Job drawing, mm, ordinate dimensions from the low corner. One solid piece. Give positions to 0.01 mm unless a question says otherwise; leave off trailing zeros. Order: outer loops, then holes, each group sorted by start corner. A loop starts at its lowest first (then second) coordinate and runs counter-clockwise, first axis right, second up.
1. Slice it at B-B on x = 84. List the corners of the cut face in (y, z), and give its area (3 significant figures).
2. Slice it at A-A on y = 57.5. List the corners of the cut face in (x, z).
3. Drop flat-ended pins along their axis: pin 1 Ø5 at (x, y) = (88.5, 47) entering from -Z; pin 2 Ø1.8 at (x, y) = (139.69, 10.87) entering from +Z. Give the stop position or say it passes through.
4. Slice it at C-C on z = 4. List the corners of the cut face in (x, y), and give its area (3 significant figures).
5. Probe line 1 (X direction, y = 87.5, z = 1.55); line 2 (Y direction, x = 8, z = 4.5) (1 decimal). List the from-to ranges inside material, lowest first.
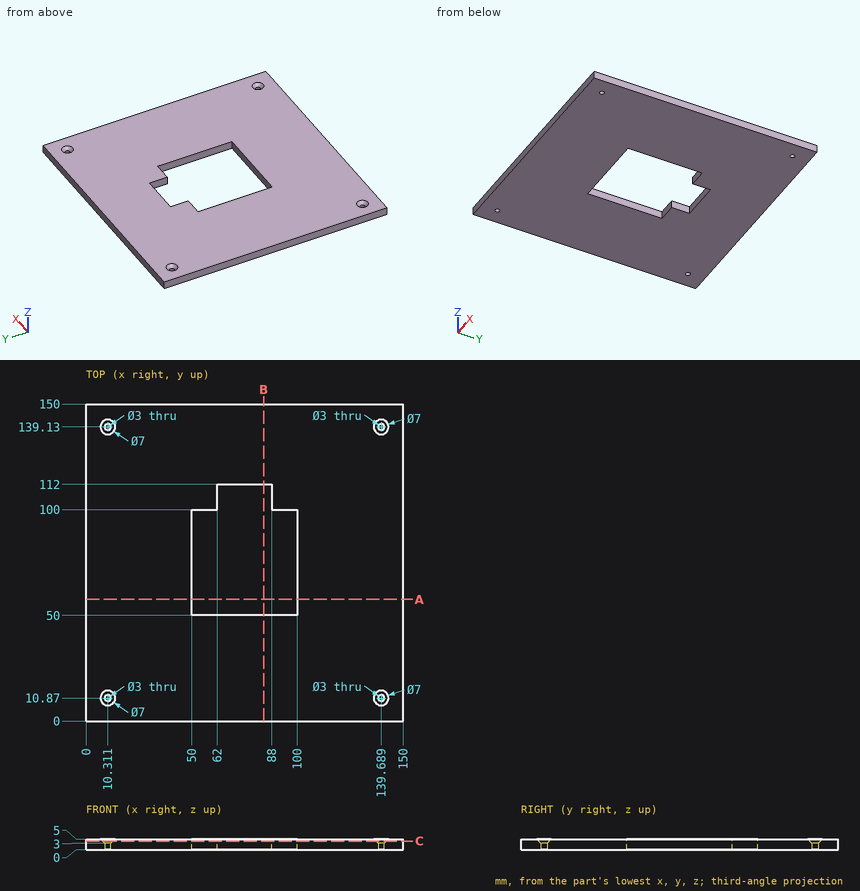
Data:
1. outline: (0, 0) - (50, 0) - (50, 5) - (0, 5) - close; (112, 0) - (150, 0) - (150, 5) - (112, 5) - close
1. area: 440 mm2
2. outline: (0, 0) - (50, 0) - (50, 5) - (0, 5) - close; (100, 0) - (150, 0) - (150, 5) - (100, 5) - close
3. pin 1: stops at z = 0
3. pin 2: passes through
4. outline: (0, 0) - (150, 0) - (150, 150) - (0, 150) - close; hole circle Ø5 at (10.31, 10.87); hole circle Ø5 at (10.31, 139.13); hole (50, 50) - (100, 50) - (100, 100) - (88, 100) - (88, 112) - (62, 112) - (62, 100) - (50, 100) - close; hole circle Ø5 at (139.69, 10.87); hole circle Ø5 at (139.69, 139.13)
4. area: 19,600 mm2
5. line 1: x = 0 to 50, 100 to 150
5. line 2: y = 0 to 9, 12.8 to 137.2, 141 to 150
